Verification items for the finished model (mm, model axes). A direction names the side the tool comes from. Round coordinates to 2 decimals unless told otherwise and drop trailing zeros. Loops run counter-clockwise (first coordinate to the right, second up) from the corner with the lowest first, then second, coordinate; pieces in that order, holes last. Notation, with made-up numbers: (78.25, 7.5) - (113.25, 7.5) arc R34 ccw to (113.25, 38.5) - close; hole circle Ø11 at (59, 17). An arc over 180 degrees is marked (long way). Use CSV: the item, a comma, the result in double quotes.
```python
from build123d import *

# Parameters (mm, degrees)
EXTRUDE_1_DEPTH     = 16
CUT_EXTRUDE_1_DEPTH = 29
FILLET_1_R          = 3
SKETCH_3_R          = 1.7
CUT_EXTRUDE_2_DEPTH = 16
SKETCH_4_R          = 2.2
CUT_EXTRUDE_3_DEPTH = 3.0606
CUT_EXTRUDE_4_DEPTH = 3
EXTRUDE_START       = 13
SKETCH_6_W          = 8
SKETCH_6_H          = 8
SKETCH_6_R          = 1.7
EXTRUDE_2_DEPTH     = 13
SKETCH_8_W          = 39.2
SKETCH_8_H          = 19.2
EXTRUDE_3_DEPTH     = 6
SKETCH_9_W          = 41.779638264
SKETCH_9_H          = 22.131707322
CUT_EXTRUDE_5_DEPTH = 45.001818144


with BuildPart() as part:
    # Эскиз1 → Бобышка-Вытянуть1 (new body)
    with BuildSketch(Plane.XY):
        Polygon((8, -16), (-8, -16), (-8, -20), (-16, -20), (-16, -16), (-16, 16), (16, 16), (16, -16), (16, -20), (8, -20), align=None)
    extrude(amount=EXTRUDE_1_DEPTH)

    # Эскиз2 → Вырез-Вытянуть1 (cut)
    with BuildSketch(Plane(origin=(0, 16, 0), x_dir=(1, 0, 0), z_dir=(0, 1, 0))):
        with BuildLine():
            Line((5.1, -11), (-5.1, -11))
            ThreePointArc((-5.1, -11), (-7.928427125, -9.828427125), (-9.1, -7))
            Line((-9.1, -7), (-9.1, -5.8))
            ThreePointArc((-9.1, -5.8), (-7.928427125, -2.971572875), (-5.1, -1.8))
            Line((-5.1, -1.8), (5.1, -1.8))
            ThreePointArc((5.1, -1.8), (7.928427125, -2.971572875), (9.1, -5.8))
            Line((9.1, -5.8), (9.1, -7))
            ThreePointArc((9.1, -7), (7.928427125, -9.828427125), (5.1, -11))
        make_face()
    extrude(amount=-CUT_EXTRUDE_1_DEPTH, mode=Mode.SUBTRACT)

    # Скругление1
    fillet_1_edges = [part.edges().sort_by_distance(p)[0] for p in [
        (7.928427125, -13, 2.971572875),
        (9.1, -13, 6.4),
        (7.928427125, -13, 9.828427125),
        (0, -13, 11),
        (-7.928427125, -13, 9.828427125),
        (-9.1, -13, 6.4),
        (-7.928427125, -13, 2.971572875),
        (0, -13, 1.8),
    ]]
    fillet(fillet_1_edges, radius=FILLET_1_R)

    # Эскиз3 → Вырез-Вытянуть2 (cut)
    with BuildSketch(Plane(origin=(0, 0, 0), x_dir=(-1, 0, 0), z_dir=(0, 0, -1))):
        with Locations((-12, -16)):
            Circle(SKETCH_3_R)
        with Locations((-12, 5)):
            Circle(SKETCH_3_R)
        with Locations(Location((12, 5, 0), (0, 0, 180))):
            Circle(SKETCH_3_R)
        with Locations(Location((12, -16, 0), (0, 0, 180))):
            Circle(SKETCH_3_R)
    extrude(amount=-CUT_EXTRUDE_2_DEPTH, mode=Mode.SUBTRACT)

    # Эскиз4 → Вырез-Вытянуть3 (cut)
    with BuildSketch(Plane(origin=(0, -16, 0), x_dir=(1, 0, 0), z_dir=(0, 1, 0))):
        with Locations(Location((0, -6.4, 0), (0, 0, 133.341758227))):
            Circle(SKETCH_4_R)
    extrude(amount=CUT_EXTRUDE_3_DEPTH, mode=Mode.SUBTRACT)

    # Эскиз5 → Вырез-Вытянуть4 (cut)
    with BuildSketch(Plane.XY.offset(16)):
        Polygon((-12, -12.709103466), (-14.85, -14.354551733), (-14.85, -17.645448267), (-12, -19.290896534), (-9.15, -17.645448267), (-9.15, -14.354551733), align=None)
        Polygon((9.15, -14.354551733), (12, -12.709103466), (14.85, -14.354551733), (14.85, -17.645448267), (12, -19.290896534), (9.15, -17.645448267), align=None)
    extrude(amount=-CUT_EXTRUDE_4_DEPTH, mode=Mode.SUBTRACT)

    # Эскиз6 → Бобышка-Вытянуть2 (add)
    # profile 1 of 2: a face of its own
    with BuildSketch(Plane(origin=(0, 0, 0), x_dir=(-1, 0, 0), z_dir=(0, 0, -1)).offset(EXTRUDE_START)):
        with Locations((-12, -16)):
            Rectangle(SKETCH_6_W, SKETCH_6_H)
        with Locations((-12, -16)):
            Circle(SKETCH_6_R, mode=Mode.SUBTRACT)
    # profile 2 of 2: a face of its own
    with BuildSketch(Plane(origin=(0, 0, 0), x_dir=(-1, 0, 0), z_dir=(0, 0, -1)).offset(EXTRUDE_START)):
        with Locations((12, -16)):
            Rectangle(SKETCH_6_W, SKETCH_6_H)
        with Locations(Location((12, -16, 0), (0, 0, 180))):
            Circle(SKETCH_6_R, mode=Mode.SUBTRACT)
    extrude(amount=-EXTRUDE_2_DEPTH)

    # Эскиз8 → Бобышка-Вытянуть3 (add)
    with BuildSketch(Plane(origin=(0, 16, 0), x_dir=(1, 0, 0), z_dir=(0, 1, 0))):
        with Locations((0, -6.4)):
            Rectangle(SKETCH_8_W, SKETCH_8_H)
        with BuildLine():
            Line((-9.1, -5.8), (-9.1, -7))
            ThreePointArc((-9.1, -7), (-7.928427125, -9.828427125), (-5.1, -11))
            Line((-5.1, -11), (5.1, -11))
            ThreePointArc((5.1, -11), (7.928427125, -9.828427125), (9.1, -7))
            Line((9.1, -7), (9.1, -5.8))
            ThreePointArc((9.1, -5.8), (7.928427125, -2.971572875), (5.1, -1.8))
            Line((5.1, -1.8), (-5.1, -1.8))
            ThreePointArc((-5.1, -1.8), (-7.928427125, -2.971572875), (-9.1, -5.8))
        make_face(mode=Mode.SUBTRACT)
    extrude(amount=-EXTRUDE_3_DEPTH)

    # Эскиз9 → Вырез-Вытянуть5 (cut, through all)
    with BuildSketch(Plane(origin=(0, 16, 0), x_dir=(1, 0, 0), z_dir=(0, 1, 0))):
        with Locations((1.289819132, 4.665853661)):
            Rectangle(SKETCH_9_W, SKETCH_9_H)
    extrude(amount=-CUT_EXTRUDE_5_DEPTH, mode=Mode.SUBTRACT)


solid = part.part
```
1) Mould release check, pull along X, two halves, no side actions. Record for faces 1 (the face through (-19.6, 13, 11)), 2 (the face through (-0.07, -12.1, 10.14)), 3 (the face through (-13, -2, 6.4)): +X half, -X half, draft (parallel to the pull), parting line (faces both ways), or undercut.
Returned:
face 1,"-X half"
face 2,"undercut"
face 3,"draft"
2) Cross-section at D-D, the plane y = -5.5. Record the cut outline in (x, z).
Returned:
outline,"(-16, 6.4) - (-9.1, 6.4) - (-9.1, 7) arc R4 cw to (-5.1, 11) - (5.1, 11) arc R4 cw to (9.1, 7) - (9.1, 6.4) - (16, 6.4) - (16, 16) - (-16, 16) - close"
3) Cross-section at C-C, the plane x = -3. Record the cut outline in (y, z).
Returned:
outline,"(-16, 6.4) - (-13, 6.4) - (-13, 8) arc R3 cw to (-10, 11) - (16, 11) - (16, 16) - (-16, 16) - close"
4) Cross-section at B-B, the plane z = 12. Record the cut outline in (x, y).
Returned:
outline,"(-19.6, 10) - (-16, 10) - (-16, -20) - (-8, -20) - (-8, -16) - (8, -16) - (8, -20) - (16, -20) - (16, 10) - (19.6, 10) - (19.6, 16) - (-19.6, 16) - close; hole circle Ø3.4 at (-12, -16); hole circle Ø3.4 at (-12, 5); hole circle Ø3.4 at (12, -16); hole circle Ø3.4 at (12, 5)"
5) Gauge pin test, flat ends, axial feed: pin 1 Ø0.8 at (x, z) = (-4.5, 7.5) entering from +Y; pin 2 Ø4 at (x, y) = (9, -2.5) entering from -Z; pin 3 Ø3.5 at (y, z) = (-16, 15) entering from +X; pin 4 Ø5.5 at (x, y) = (-12, -16) entering from +Z. Record the tip position at first contact, or that the pin passes through.
Returned:
pin 1,"stops at y = -13"
pin 2,"stops at z = 6.4"
pin 3,"stops at x = 16"
pin 4,"stops at z = 13"
6) Thickness scan on probe 1 along Y at (x, z) = (12, 12.5); probe 2 along X at (y, z) = (-16.5, 9.5); probe 3 along Z at (x, y) = (0, 14). Record the ranges inside material, lowest first. Write a range as [from, to].
Returned:
probe 1,"y = [-20, -17.7], [-14.3, 3.3], [6.7, 16]"
probe 2,"x = [-16, -13.62], [-10.38, -8], [8, 10.38], [13.62, 16]"
probe 3,"z = [11, 16]"
7) Cross-section at A-A, the plane y = 5. Record the cut outline in (x, z), then the cut area to 3 significant figures.
Returned:
outline,"(-16, 6.4) - (-13.7, 6.4) - (-13.7, 16) - (-16, 16) - close; (-10.3, 6.4) - (-9.1, 6.4) - (-9.1, 7) arc R4 cw to (-5.1, 11) - (5.1, 11) arc R4 cw to (9.1, 7) - (9.1, 6.4) - (10.3, 6.4) - (10.3, 16) - (-10.3, 16) - close; (13.7, 6.4) - (16, 6.4) - (16, 16) - (13.7, 16) - close"
area,"165 mm²"
8) Access from +Z, -Z, +X, -X, +Y, -Y to the whole of each face (thin tool, end or side, straight path). Record for faces 4 (the face through (8.24, -12.1, 6.7)), 5 (the face through (18, 10, 11)), 6 (the face through (-14.85, -16, 15)), 7 (the face through (0, -14.5, 8.6)), 8 (the face through (8, -18, 11)).
Returned:
face 4,"-Z, +Y"
face 5,"+Z, -Z, +X, -Y"
face 6,"+Z"
face 7,"-Z, +Y, -Y"
face 8,"+Z, -Z, -Y"
